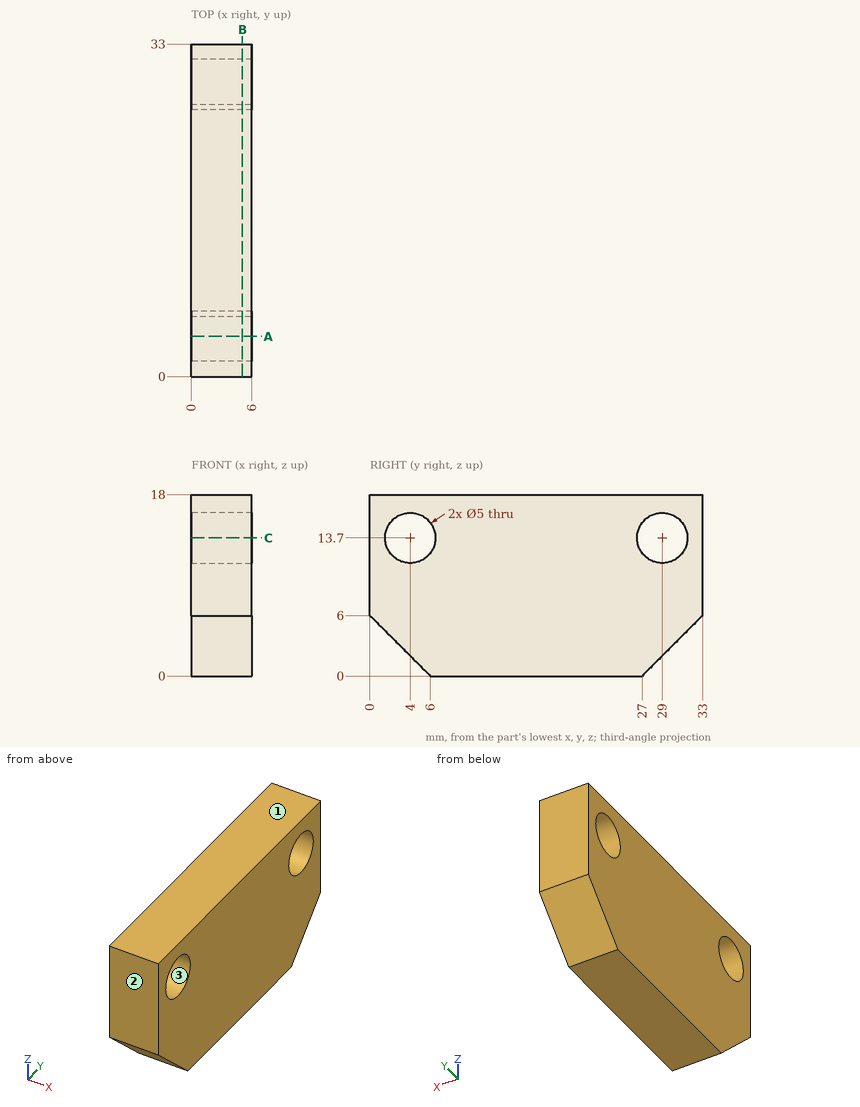
Print and shaded views of the part. All mm, measured from the part's lowest x, y and z. Round coordinates to 2 decimals unless told otherwise and drop trailing zeros. Write each loop counter-clockwise with the first axis right and the second up, starting at its lowest first coordinate (ties: lowest second). Pieces come first, ordered by that corner, then holes.
Item 1: Cut at A-A, the plane y = 4. Give the cut face in (x, z), plus the area to 3 significant figures.
Results:
outline: (0, 2) - (6, 2) - (6, 11.2) - (0, 11.2) - close; (0, 16.2) - (6, 16.2) - (6, 18) - (0, 18) - close
area: 66.0 mm2
Item 2: Cut at B-B, the plane x = 5.05. Give the cut face in (y, z), plus the area to 3 significant figures.
Results:
outline: (0, 6) - (6, 0) - (27, 0) - (33, 6) - (33, 18) - (0, 18) - close; hole circle Ø5 at (4, 13.7); hole circle Ø5 at (29, 13.7)
area: 519 mm2
Item 3: Cut at C-C, the plane z = 13.7. Give the cut face in (x, y).
Results:
outline: (0, 0) - (6, 0) - (6, 1.5) - (0, 1.5) - close; (0, 6.5) - (6, 6.5) - (6, 26.5) - (0, 26.5) - close; (0, 31.5) - (6, 31.5) - (6, 33) - (0, 33) - close
Item 4: Two-plate mould, pull along Y, no slides. Class the marked faces 1, 2 and 3: +Y half, -Y half, draft (parallel to the pull), parting line (faces both ways), or undercut.
Results:
face 1: draft
face 2: -Y half
face 3: undercut
Item 5: Probe L1, parallel to Y at x = 1.8, z = 13.7; L2, parallel to Y at x = 2.9, z = 14.5; L3, parallel to Z at x = 3.2, y = 29. List the from-to ranges inside material, lowest first.
Results:
L1: y = 0 to 1.5, 6.5 to 26.5, 31.5 to 33
L2: y = 0 to 1.63, 6.37 to 26.63, 31.37 to 33
L3: z = 2 to 11.2, 16.2 to 18
